```python
from build123d import *

# Parameters (mm, degrees)
ESQUISSE1_R        = 1
ESQUISSE1_R_2      = 1.75
BOSS_EXTRU_1_DEPTH = 2


with BuildPart() as part:
    # Esquisse1 → Boss.-Extru.1 (new body)
    with BuildSketch(Plane(origin=(-102.847426705, 0, 18.134776225), x_dir=(-0.9358900387216226, 0, 0.3522922585320884), z_dir=(0, -1, 0))):
        with BuildLine():
            Line((-29.681110437, -6.92992201), (-25.193077168, -6.601962606))
            ThreePointArc((-25.193077168, -6.601962606), (-31.376531627, 14.125140597), (-45.701784247, 30.331159651))
            ThreePointArc((-45.701784247, 30.331159651), (-46.468142588, 35.221220478), (-41.578081761, 35.987578819))
            ThreePointArc((-41.578081761, 35.987578819), (-34.948662945, 30.333854293), (-29.254192772, 23.739401754))
            ThreePointArc((-29.254192772, 23.739401754), (-22.67424344, 20.714879645), (-16.604130615, 24.664208385))
            ThreePointArc((-16.604130615, 24.664208385), (-11.931476736, 32.014751147), (-6.198466062, 38.571942755))
            ThreePointArc((-6.198466062, 38.571942755), (-1.248925128, 38.526726063), (-1.294141821, 33.577185129))
            ThreePointArc((-1.294141821, 33.577185129), (-13.111349847, 15.448077308), (-16.215278728, -5.968658704))
            Line((-16.215278728, -5.968658704), (-11.727259944, -5.640718208))
            ThreePointArc((-11.727259944, -5.640718208), (-8.820974111, -6.603051654), (-7.446392196, -9.338578579))
            Line((-7.446392196, -9.338578579), (-6.571881132, -21.306670758))
            ThreePointArc((-6.571881132, -21.306670758), (-7.534214578, -24.212956591), (-10.269741503, -25.587538506))
            Line((-10.269741503, -25.587538506), (-14.757760288, -25.915479002))
            ThreePointArc((-14.757760288, -25.915479002), (-15.331661084, -40.585109619), (-17.13310324, -55.155018018))
            ThreePointArc((-17.13310324, -55.155018018), (-20.734362801, -40.921154617), (-23.735479814, -26.548777137))
            Line((-23.735479814, -26.548777137), (-28.223513084, -26.876736542))
            ThreePointArc((-28.223513084, -26.876736542), (-31.129802724, -25.914414593), (-32.504395461, -23.178893106))
            Line((-32.504395461, -23.178893106), (-33.378953873, -11.210804387))
            ThreePointArc((-33.378953873, -11.210804387), (-32.416631925, -8.304514747), (-29.681110437, -6.92992201))
        make_face()
        with Locations(Location((-43.639933004, 33.159369235, 0), (0, 0, 110.627584138))):
            Circle(ESQUISSE1_R, mode=Mode.SUBTRACT)
        with Locations(Location((-29.389590967, -10.919284916, 0), (0, 0, 110.627584138))):
            Circle(ESQUISSE1_R_2, mode=Mode.SUBTRACT)
        with Locations(Location((-28.515032555, -22.887373635, 0), (0, 0, 110.627584138))):
            Circle(ESQUISSE1_R_2, mode=Mode.SUBTRACT)
        with Locations(Location((-10.561245191, -21.598174446, 0), (0, 0, 110.627584138))):
            Circle(ESQUISSE1_R_2, mode=Mode.SUBTRACT)
        with Locations(Location((-11.435756256, -9.630082268, 0), (0, 0, 110.627584138))):
            Circle(ESQUISSE1_R_2, mode=Mode.SUBTRACT)
        with Locations(Location((-3.746303941, 36.074563942, 0), (0, 0, 110.627584138))):
            Circle(ESQUISSE1_R, mode=Mode.SUBTRACT)
    extrude(amount=BOSS_EXTRU_1_DEPTH)


solid = part.part
```
Geometry check sheet. Reference: the model listing, model coordinates, mm. A direction names the side the tool comes from. Coordinates: 2 decimals unless noted, no trailing zeros. Loops run counter-clockwise (first coordinate to the right, second up) from the corner with the lowest first, then second, coordinate; pieces in that order, holes last. Notation, with made-up numbers: (68.5, 10.5) - (100.5, 10.5) arc R18 cw to (100.5, 36.5) - close; hole circle Ø11 at (10, 26.5). An arc over 180 degrees is marked (long way). One line per item, written item: value. Start each with the question number.
(1) Cross-section at D-D on x = -103. Enter the section's corners in (y, z).
(2) Tool access check on faces 1 (the flat face through (-74.756, -0.986, 14.792)), 2 (the cylindrical face through (-69, -0.99, 49.33)), 3 (the flat face through (-82.094, -0.986, 37.836)). Record the directions out of +Z, -Z, +X, -X, +Y, -Y that give a thin tool (end or side, any length) a straight path to the whole face; none if there is none.
(3) Cross-section at C-C on z = 13. Enter the section's corners in (x, y), plus the area to 3 significant figures.
(4) Material ranges on line 1 (Z direction, x = -88, y = -0.05); line 2 (Z direction, x = -73, y = -1.5); line 3 (X direction, y = -1.8, z = -28), recorded low to high. Write a range as [from, to].
(5) Depth check by flat-ended pin: P1, Ø1.8, axis at x = -112.05, z = -16.95, coming from the -Y side. Enter the tip coordinate at first touch or a pass-through.
(6) Cross-section at A-A on y = -1.5. Enter the section's corners in (x, z).
(7) Mould release check, pull along Z, two halves, no side actions. Record for faces 4 (the cylindrical face through (-69.65, -0.99, 28.7)), 5 (the cylindrical face through (-80.775, -0.986, -22.678)), 6 (the cylindrical face through (-96.22, -0.99, -1.17)), 7 (the cylindrical face through (-87.305, -0.986, 38.12)): released by +Z, released by -Z, zero draft, split by the parting line, or undercut.
(8) Cross-section at B-B on z = 30. Enter the section's corners in (x, y).
Results below:
1. outline: (-2, -16.06) - (0, -16.06) - (0, -7.51) - (-2, -7.51) - close
2. face 1: +Y, -Y
2. face 2: +X, +Y, -Y
2. face 3: +Z, +Y, -Y
3. outline: (-87.34, -2) - (-77.6, -2) - (-77.6, 0) - (-87.34, 0) - close
3. area: 19.5 mm2
4. line 1: z = [-9.58, 11.48], [18.73, 21.54], [24.7, 37.63]
4. line 2: z = [-31.7, -29], [-27.55, -22.59], [14.27, 17.11], [18.89, 53.21]
4. line 3: x = [-77.98, -74.65], [-72.72, -70.2]
5. P1: passes through
6. outline: (-113.47, -13.75) arc R3.5 ccw to (-110.63, -20.15) arc R57.29 ccw to (-96, -10.8) arc R7.5 cw to (-83.83, -14.39) arc R57.24 ccw to (-76.61, -30.19) arc R3.5 ccw to (-70.76, -26.35) arc R50.24 cw to (-76.94, 15.44) - (-72.63, 14.16) arc R4 ccw to (-67.66, 16.87) - (-64.26, 28.38) arc R4 ccw to (-66.96, 33.35) - (-71.28, 34.62) arc R350 ccw to (-67.38, 63.72) arc R175 ccw to (-79.91, 37.19) - (-84.22, 38.46) arc R4 ccw to (-89.19, 35.76) - (-92.59, 24.25) arc R4 ccw to (-89.88, 19.28) - (-85.57, 18.01) arc R50.29 cw to start; hole circle Ø2 at (-112.05, -16.95); hole circle Ø3.5 at (-88.75, 23.12); hole circle Ø3.5 at (-85.35, 34.63); hole circle Ø2 at (-73.69, -28.27); hole circle Ø3.5 at (-71.5, 18); hole circle Ø3.5 at (-68.1, 29.51)
7. face 4: undercut
7. face 5: released by -Z
7. face 6: undercut
7. face 7: released by +Z
8. outline: (-90.89, -2) - (-69.78, -2) - (-69.78, 0) - (-90.89, 0) - close; (-66.42, -2) - (-64.13, -2) - (-64.13, 0) - (-66.42, 0) - close
